Check sheet for the modelled part. Datum: model origin and axes. Units: mm. A direction names the side the tool comes from. Round coordinates to 2 decimals unless told otherwise and drop trailing zeros. Loops run counter-clockwise (first coordinate to the right, second up) from the corner with the lowest first, then second, coordinate; pieces in that order, holes last. Notation, with made-up numbers: (71.5, -32) - (119.5, -32) arc R17 cw to (119.5, -1) - close; hole circle Ø4 at (65.25, -23). An arc over 180 degrees is marked (long way). Put each result on its own line as item: value. Start each with the question number.
Item 1: Section check D-D, the plane x = -3. Record the cut outline in (y, z), and give its area (3 significant figures).
Item 2: Section check C-C, the plane y = 15. Record the cut outline in (x, z).
Item 3: Gauge pin test, flat ends, axial feed: pin 1 Ø5 at (x, y) = (2.5, 5) entering from +Z; pin 2 Ø6 at (y, z) = (-2, -0.5) entering from +X. Record the tip position at first contact, or that the pin passes through.
Item 4: Section check B-B, the plane z = 2.5. Record the cut outline in (x, y), and give its area (3 significant figures).
Item 5: Section check A-A, the plane x = 0. Record the cut outline in (y, z), and give its area (3 significant figures).
Item 6: Material ranges on line 1 along Z through (x, y) = (0, -4.5); line 2 along X through (y, z) = (-7, 2.5); line 3 along Y through (x, z) = (-4.5, 0.75), recorded low to high.
Item 7: Tool access check on faces 1 (the flat face through (0, 0, 2.5)), 2 (the flat face through (-4, 42, 5)), 3 (the cylindrical face through (4.88, 21.29, 3.58)). Record the directions out of +Z, -Z, +X, -X, +Y, -Y that give a thin tool (end or side, any length) a straight path to the whole face; none if there is none.
Solid Edge part; units mm, degrees
sketch "Sketch1" plane through (0, 0, 0) normal (-1, 0, 0) x (0, -1, 0)
  line L0 (0, 2.5) -> (-42, 2.5)
  line L1 (-42, 2) -> (-42, 2.5)
  line L2 (-42, 2) -> (-51, 2)
  line L3 (-51, 2) -> (-51, -2)
  line L4 (-42, -2) -> (-51, -2)
  line L5 (-42, -2.5) -> (-42, -2)
  line L6 (0, -2.5) -> (-42, -2.5)
  line L7 (0, -2) -> (0, -2.5)
  line L8 (9, -2.001) -> (0, -2)
  line L9 (9, 2) -> (9, -2.001)
  line L10 (0, 2) -> (9, 2)
  line L11 (0, 2.5) -> (0, 2)
revolve "RevolvedProtrusion1" add sketch "Sketch1" angle 360 about axis through (0, 0, 2.5) along (0, 1, 0)
Check result:
1. outline: (-9, -0.86) - (0, -0.86) - (0, -1.5) - (42, -1.5) - (42, -0.85) - (51, -0.85) - (51, 5.85) - (42, 5.85) - (42, 6.5) - (0, 6.5) - (0, 5.85) - (-9, 5.86) - close
1. area: 457 mm²
2. outline: circle Ø10 at (0, 2.5)
3. pin 1: z = 7.5
3. pin 2: x = 4.94
4. outline: (-5, 0) - (-4.5, 0) - (-4.5, -9) - (-0.5, -9) - (-0.5, 0) - (0.5, 0) - (0.5, -9) - (4.5, -9) - (4.5, 0) - (5, 0) - (5, 42) - (4.5, 42) - (4.5, 51) - (0.5, 51) - (0.5, 42) - (-0.5, 42) - (-0.5, 51) - (-4.5, 51) - (-4.5, 42) - (-5, 42) - close
4. area: 564 mm²
5. outline: (-9, -2) - (0, -2) - (0, -2.5) - (42, -2.5) - (42, -2) - (51, -2) - (51, 2) - (42, 2) - (42, 3) - (51, 3) - (51, 7) - (42, 7) - (42, 7.5) - (0, 7.5) - (0, 7) - (-9, 7) - (-9, 3) - (0, 3) - (0, 2) - (-9, 2) - close
5. area: 564 mm²
6. line 1: -2 to 2, 3 to 7
6. line 2: -4.5 to -0.5, 0.5 to 4.5
6. line 3: 0 to 42
7. face 1: -Y
7. face 2: +Y
7. face 3: +Y, -Y
